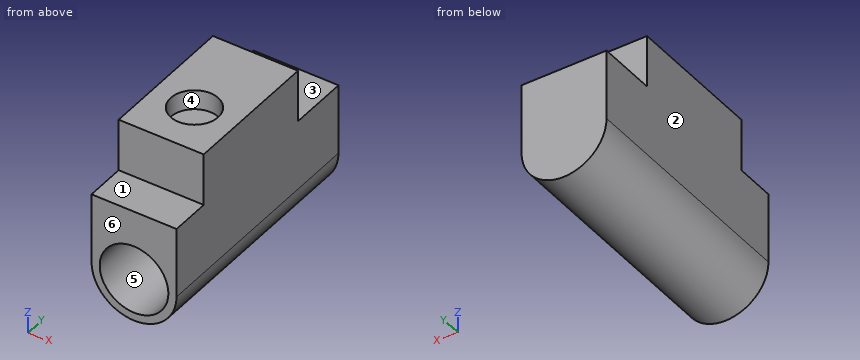
Autodesk Inventor part; units mm, degrees
ref_plane "YZ Plane" through (0, 0, 0) normal (1, 0, 0) x (0, 1, 0)
ref_plane "XZ Plane" through (0, 0, 0) normal (0, 1, 0) x (-1, 0, 0)
ref_plane "XY Plane" through (0, 0, 0) normal (0, 0, 1) x (1, 0, 0)
sketch "Sketch1" plane through (0, 0, 0) normal (0, 0, 1) x (1, 0, 0)
  circle A0 centre (0, 0) radius 18.4404
  line L0 (-33.02, -38.1) -> (33.02, -38.1)
  line L1 (33.02, -38.1) -> (33.02, 69.85)
  line L2 (33.02, 69.85) -> (-33.02, 69.85)
  line L3 (-33.02, 69.85) -> (-33.02, -38.1)
  dimension "d0" = 36.8808
  dimension "d1" = 66.04
  dimension "d2" = 107.95
  dimension "d3" = 33.02
  dimension "d4" = 38.1
extrude "Extrusion1" add sketch "Sketch1" against normal blind 40.64
sketch "Sketch2" plane through (0, 0, -40.64) normal (0, 0, -1) x (-1, 0, 0)
  circle A0 centre (0, 0) radius 25.1006
extrude "Extrusion2" add sketch "Sketch2" against normal blind 25.4
sketch "Sketch3" plane through (-33.02, -38.1, 0) normal (0, -1, 0) x (1, 0, 0)
  line L0 (0, 0) -> (66.04, 0)
  line L1 (66.04, 0) -> (0, 0)
  line L2 (0, 0) -> (0, -95.25)
  line L3 (0, -95.25) -> (66.04, -95.25)
  line L4 (66.04, -95.25) -> (66.04, 0)
  line L5 (66.04, -40.64) -> (0, -40.64)
  arc A0 (0, -95.25) -> (66.04, -95.25) centre (33.02, -95.25) ccw
  line L6 (0, -40.64) -> (66.04, -40.64)
  line L7 (0, -40.64) -> (66.04, -40.64)
  line L8 (66.04, -40.64) -> (66.04, -95.25)
  line L9 (66.04, -95.25) -> (0, -95.25)
  line L10 (0, -95.25) -> (0, -40.64)
  point P0 (33.02, 0)
  dimension "d9" = 54.61
extrude "Extrusion3" add sketch "Sketch3" along normal mid plane 62.23 contours L5 L4 L3 L2 | L3 A0
sketch "Sketch4" plane through (-33.02, -38.1, 0) normal (0, -1, 0) x (1, 0, 0)
  point P0 (33.02, 0)
sketch "Sketch5" plane through (-33.02, -6.985, 0) normal (0, 1, 0) x (1, 0, 0)
  arc A0 (66.04, 95.25) -> (0, 95.25) centre (33.02, 95.25) ccw
  line L0 (66.04, 40.64) -> (66.04, 95.25)
  line L1 (0, 95.25) -> (66.04, 95.25)
  line L2 (66.04, 95.25) -> (66.04, 40.64)
  line L3 (66.04, 40.64) -> (0, 40.64)
  line L4 (0, 40.64) -> (0, 95.25)
  arc A1 (66.04, 95.25) -> (0, 95.25) centre (33.02, 95.25) ccw
  point P0 (33.02, 0)
extrude "Extrusion4" add sketch "Sketch5" along normal blind 123.19
sketch "Sketch6" plane through (-33.02, -69.215, 0) normal (0, -1, 0) x (1, 0, 0)
  arc A0 (0, -95.25) -> (66.04, -95.25) centre (33.02, -95.25) ccw
  line L0 (0, -95.25) -> (33.02, -95.25)
  circle A1 centre (33.02, -95.25) radius 26.67
  point P0 (33.02, 0)
  dimension "d16" = 53.34
extrude "Extrusion5" cut sketch "Sketch6" against normal blind 60.96
properties part number "Wrist1"
Source: CAD feature listing. Evaluate the final solid. Frame: model axes, mm. Face numbers are marked on the shaded views. A direction names the side the tool comes from. Round coordinates to 2 decimals unless told otherwise and drop trailing zeros. Loops run counter-clockwise (first coordinate to the right, second up) from the corner with the lowest first, then second, coordinate; pieces in that order, holes last. Notation, with made-up numbers: M 3.5,26.25 L 54.5,26.25 A24 cw 54.5,53.25 Z; hole C -8,53 d10. An arc over 180 degrees is marked long. Return JSON: item names as keys, results as strings. Group by question number.
1. Pin query (flat end, axial travel): pin 1 (23 mm diameter, centred on x = -10, y = 90, fed in from +Z); pin 2 (3 mm diameter, centred on x = 0, z = -37.5, fed in from +Y); pin 3 (18.5 mm diameter, centred on x = 5, y = -7, fed in from +Z). Return the tip coordinate at first contact, or that it passes through.
2. Mould query, pull axis Y, two halves, no side actions, for the marked faces 4, 5 and 6. Classes: released by +Y, released by -Y, zero draft, split by the parting line, or undercut.
3. Section query D-D on z = -89.5. Output: boundary loops of the cut face in (x, y) (3 decimals).
4. Reachability of the marked faces 1, 2 and 3 from +Z, -Z, +X, -X, +Y, -Y: full face, straight path, thin tool, end or side. Return the list, or none.
5. Section query C-C on z = -10. Output: boundary loops of the cut face in (x, y).
6. Section query A-A on y = 0. Output: boundary loops of the cut face in (x, z).
7. Material intervals for line 1 along Z through (x, y) = (0, -44); line 2 along Z through (x, y) = (0, -37); line 3 along X through (y, z) = (-50, -95), sorted ascending. Write a range as from..to.
8. Section query B-B on x = 0. Output: boundary loops of the cut face in (y, z) (3 decimals).
Checks:
{
 "1": {"pin 1": "stops at z = -40.64", "pin 2": "stops at y = 69.85", "pin 3": "stops at z = -15.24"},
 "2": {"face 4": "undercut", "face 5": "zero draft", "face 6": "released by -Y"},
 "3": {"outline": "M -33.02,-69.215 L -26.043,-69.215 L -26.043,-8.255 L 26.043,-8.255 L 26.043,-69.215 L 33.02,-69.215 L 33.02,116.205 L -33.02,116.205 Z"},
 "4": {"face 1": "+Z, +X, -X, -Y", "face 2": "+Z, -Z, -X, +Y, -Y", "face 3": "+Z, +X, -X, +Y"},
 "5": {"outline": "M -33.02,-38.1 L 33.02,-38.1 L 33.02,69.85 L -33.02,69.85 Z; hole C 0,0 d36.88"},
 "6": {"outline": "M -33.02,-95.25 A33.02 ccw 33.02,-95.25 L 33.02,0 L 18.44,0 L 18.44,-15.24 L -18.44,-15.24 L -18.44,0 L -33.02,0 Z"},
 "7": {"line 1": "z = -128.27..-121.92, -68.58..-40.64", "line 2": "z = -128.27..-121.92, -68.58..0", "line 3": "x = -33.02..-26.67, 26.67..33.02"},
 "8": {"outline": "M -69.215,-128.27 L 116.205,-128.27 L 116.205,-40.64 L 69.85,-40.64 L 69.85,0 L 18.44,0 L 18.44,-15.24 L -18.44,-15.24 L -18.44,0 L -38.1,0 L -38.1,-40.64 L -69.215,-40.64 L -69.215,-68.58 L -8.255,-68.58 L -8.255,-121.92 L -69.215,-121.92 Z"}
}
